```python
from build123d import *

# Parameters (mm, degrees)
SKETCH_1_W      = 23
SKETCH_1_H      = 54
EXTRUDE_1_DEPTH = 5
EXTRUDE_2_DEPTH = 3
SKETCH_3_W      = 55
SKETCH_3_H      = 85
EXTRUDE_3_DEPTH = 8


with BuildPart() as part:
    # 草图1 → 凸台-拉伸1 (new body)
    with BuildSketch(Plane.XY):
        Rectangle(SKETCH_1_W, SKETCH_1_H)
        Polygon((0, 6), (-5.5, 0), (0, -6), (5.5, 0), align=None, mode=Mode.SUBTRACT)
    extrude(amount=EXTRUDE_1_DEPTH)

    # 草图2 → 凸台-拉伸2 (add)
    with BuildSketch(Plane.XY.offset(5)):
        Polygon((0, -6), (5.5, 0), (0, 6), (-5.5, 0), align=None)
    extrude(amount=-EXTRUDE_2_DEPTH)

    # 草图3 → 凸台-拉伸3 (add)
    with BuildSketch(Plane.XY.offset(5)):
        Rectangle(SKETCH_3_W, SKETCH_3_H)
    extrude(amount=EXTRUDE_3_DEPTH)


solid = part.part
```
Could you check a few things on this model? Use its own coordinates, in mm. A direction names the side the tool comes from. Give positions to 0.01 mm unless a question says otherwise; leave off trailing zeros. Order: outer loops, then holes, each group sorted by start corner. A loop starts at its lowest first (then second) coordinate and runs counter-clockwise, first axis right, second up.
Q1. Suppose I cut it at B-B, the plane x = -7.5. Write out the boundary of the cut face in (y, z).
Q2. I'm going to push flat-ended pins straight in: P1, Ø2.5, axis at y = 2, z = 3.5, coming from the -X side; P2, Ø2, axis at x = -17, y = 17, coming from the -Z side; P3, Ø4, axis at x = 5.5, z = 1.5, coming from the -Y side. Where does each tip first touch, or does it pass through?
Q3. Suppose I cut it at A-A, the plane z = 1. Write out the boundary of the cut face in (x, y).
Q4. We'd pull the mould along X, two halves only. Please class faces 5 (the flat face through (-2.712, 3.042, 0.986)), 6 (the flat face through (11.5, 0, 2)), 7 (the flat face through (0, 0, 2)), 8 (the flat face through (0, 1, 13)): +X half, -X half, draft (parallel to the pull), parting line (faces both ways), or undercut.
Q5. Suppose I cut it at C-C, the plane y = 25. Write out the boundary of the cut face in (x, z).
Q6. For faces 1 (the flat face through (-11.5, 0, 2)), 2 (the flat face through (0, 27, 2)), 3 (the flat face through (0, -27, 2)), 4 (the flat face through (2.712, -3.042, 0.986)), which set-ups out of +Z, -Z, +X, -X, +Y, -Y let a thin tool reach every point of the face, with its end or its side?
Q7. Suppose I cut it at D-D, the plane y = 2.5. Write out the boundary of the cut face in (x, z), and give its area (3 significant figures).
Q8. If I drill on line 1 along Z through (x, y) = (-23.5, -6); line 2 along Y through (x, z) = (-2, 3.75); line 3 along X through (y, z) = (-6, 3.25), over which ranges is the centre line in solid material (lowest first)?
Solution:
1. outline: (-42.5, 5) - (-27, 5) - (-27, 0) - (27, 0) - (27, 5) - (42.5, 5) - (42.5, 13) - (-42.5, 13) - close
2. P1: stops at x = -11.5
2. P2: stops at z = 5
2. P3: stops at y = -27
3. outline: (-11.5, -27) - (11.5, -27) - (11.5, 27) - (-11.5, 27) - close; hole (-5.5, 0) - (0, -6) - (5.5, 0) - (0, 6) - close
4. face 5: undercut
4. face 6: +X half
4. face 7: undercut
4. face 8: draft
5. outline: (-27.5, 5) - (-11.5, 5) - (-11.5, 0) - (11.5, 0) - (11.5, 5) - (27.5, 5) - (27.5, 13) - (-27.5, 13) - close
6. face 1: -Z, -X, +Y, -Y
6. face 2: -Z, +X, -X, +Y
6. face 3: -Z, +X, -X, -Y
6. face 4: -Z
7. outline: (-27.5, 5) - (-11.5, 5) - (-11.5, 0) - (-3.21, 0) - (-3.21, 2) - (3.21, 2) - (3.21, 0) - (11.5, 0) - (11.5, 5) - (27.5, 5) - (27.5, 13) - (-27.5, 13) - close
7. area: 542 mm2
8. line 1: z = 5 to 13
8. line 2: y = -27 to 27
8. line 3: x = -11.5 to 11.5
